Build history of the part. All positions in model axes, mm. Round coordinates to 2 decimals unless told otherwise and drop trailing zeros. Write each loop counter-clockwise with the first axis right and the second up, starting at its lowest first coordinate (ties: lowest second). Pieces come first, ordered by that corner, then holes. Notation, with made-up numbers: M 82,50 L 88,50 A21 cw 88,69 Z; hole C 18.5,43 d1. An arc over 180 degrees is marked long. Write item = value, one per line.
from build123d import *

# Parameters (mm, degrees)
BOSS_EXTRUDE1_DEPTH = 6.35
BOSS_EXTRUDE2_DEPTH = 6.35
CUT_EXTRUDE1_DEPTH  = 176.195383741
SKETCH4_R           = 3
CUT_EXTRUDE2_DEPTH  = 169.439588188
SKETCH5_R           = 3.81
BOSS_EXTRUDE3_DEPTH = 6.35


with BuildPart() as part:
    # Sketch1 → Boss-Extrude1 (new body)
    with BuildSketch(Plane(origin=(0, 0, 0), x_dir=(0, 0, -1), z_dir=(1, 0, 0))):
        with BuildLine():
            Line((-106.172, 0), (-62.992, 43.18))
            Line((-62.992, 43.18), (0, 43.18))
            Line((0, 43.18), (0, 40.64))
            ThreePointArc((0, 40.64), (-6.479930943, 21.59), (0, 2.54))
            Line((0, 2.54), (0, 0))
            Line((0, 0), (-106.172, 0))
        make_face()
    extrude(amount=BOSS_EXTRUDE1_DEPTH)

    # Sketch2 → Boss-Extrude2 (add)
    with BuildSketch(Plane(origin=(6.35, 0, 0), x_dir=(0, 0, -1), z_dir=(1, 0, 0))):
        Polygon((-68.072, 0), (-169.672, 0), (-144.272, 10.16), (-68.072, 17.78), align=None)
    extrude(amount=-BOSS_EXTRUDE2_DEPTH)

    # Sketch3 → Cut-Extrude1 (cut, through all)
    with BuildSketch(Plane(origin=(6.35, 0, 0), x_dir=(0, 0, -1), z_dir=(1, 0, 0))):
        Polygon((-106.172, 0), (-162.687, 2.794), (-169.672, 0), align=None)
    extrude(amount=-CUT_EXTRUDE1_DEPTH, mode=Mode.SUBTRACT)

    # Sketch4 → Cut-Extrude2 (cut, through all)
    with BuildSketch(Plane(origin=(6.35, 0, 0), x_dir=(0, 0, -1), z_dir=(1, 0, 0))):
        with Locations((-25.4, 31.59)):
            Circle(SKETCH4_R)
        with Locations((-25.4, 11.59)):
            Circle(SKETCH4_R)
        with Locations((-76.2, 11.59)):
            Circle(SKETCH4_R)
    extrude(amount=-CUT_EXTRUDE2_DEPTH, mode=Mode.SUBTRACT)

    # Sketch5 → Boss-Extrude3 (add)
    with BuildSketch(Plane.ZY):
        with BuildLine():
            Line((0, 43.18), (-43.481110833, 43.18))
            ThreePointArc((-43.481110833, 43.18), (-53.337069057, 21.59), (-43.481110833, 0))
            Line((-43.481110833, 0), (0, 0))
            Line((0, 0), (0, 2.54))
            ThreePointArc((0, 2.54), (6.479930943, 21.59), (0, 40.64))
            Line((0, 40.64), (0, 43.18))
        make_face()
        with Locations((-24.762069057, 21.59)):
            Circle(SKETCH5_R, mode=Mode.SUBTRACT)
    extrude(amount=-BOSS_EXTRUDE3_DEPTH)


solid = part.part
1. Band-saw the part on A-A (x = 3.75). List the corners of the cut face in (y, z) (3 decimals).
Responses:
outline = M 0,-43.481 A28.575 ccw 43.18,-43.481 L 43.18,62.992 L 15.522,90.65 L 10.16,144.272 L 2.794,162.687 L 0,106.172 Z; hole C 11.59,25.4 d6; hole C 11.59,76.2 d6; hole C 21.59,-24.762 d7.62; hole C 31.59,25.4 d6
2. Mould opens along Z. For faces 1 (the face through (3.22, 10.44, 22.63)), 2 (the face through (3.131, 21.933, -53.335)), 3 (the face through (3.219, 12.804, 117.836)) say: pulls with the +Z half, pulls with the -Z half, needs draft (parallel to the pull), parting line crosses it, or undercut.
Responses:
face_1 = undercut
face_2 = pulls with the -Z half
face_3 = pulls with the +Z half
3. Probe probe 1 along Y at (x, z) = (3.5, 25.4); probe 2 along Z at (x, y) = (2, 34); probe 3 along Z at (x, y) = (1.25, 23.5). List the from-to ranges inside material, lowest first.
Responses:
probe_1 = 0 to 8.59, 14.59 to 28.59, 34.59 to 43.18
probe_2 = -50.5 to 23.61, 27.19 to 72.17
probe_3 = -53.27 to -28.06, -21.47 to 82.67
4. Band-saw the part on C-C (y = 21.59). List the corners of the cut face in (x, z).
Responses:
outline = M 0,-53.34 L 6.35,-53.34 L 6.35,-28.57 L 0,-28.57 Z; M 0,-20.95 L 6.35,-20.95 L 6.35,84.58 L 0,84.58 Z
5. Band-saw the part on B-B (z = 76.2). List the corners of the cut face in (x, y).
Responses:
outline = M 0,0 L 6.35,0 L 6.35,8.59 L 0,8.59 Z; M 0,14.59 L 6.35,14.59 L 6.35,29.97 L 0,29.97 Z
6. Flat gauge pins, fed straight in: pin 1 (1 mm diameter, centred on x = 4, y = 33.5, fed in from -Z); pin 2 (4.5 mm diameter, centred on y = 21.59, z = -24.76, fed in from +X); pin 3 (1 mm diameter, centred on x = 5.5, y = 30, fed in from -Z); pin 4 (1.5 mm diameter, centred on x = 3, y = 5, fed in from +Z). Where does each tip first touch, or does it go through?
Responses:
pin_1 = -50.96
pin_2 = through
pin_3 = -52.22
pin_4 = 159.05
7. Band-saw the part on D-D (z = 25). List the corners of the cut face in (x, y), plus the area to 3 significant figures.
Responses:
outline = M 0,0 L 6.35,0 L 6.35,8.62 L 0,8.62 Z; M 0,14.56 L 6.35,14.56 L 6.35,28.62 L 0,28.62 Z; M 0,34.56 L 6.35,34.56 L 6.35,43.18 L 0,43.18 Z
area = 199 mm²
